The listing builds one solid part. Answer for the finished solid, in the listing's coordinates (mm). Give positions to 0.01 mm unless a question says otherwise; leave off trailing zeros. Write each loop counter-clockwise with the first axis right and the second up, starting at its lowest first coordinate (ties: lowest second). Pieces come first, ordered by that corner, then holes.
```python
from build123d import *

# Parameters (mm, degrees)
SKETCH1_W                        = 44.45
SKETCH1_H                        = 44.45
SKETCH1_W_2                      = 38.1
SKETCH1_H_2                      = 38.1
BOSS_EXTRUDE1_DEPTH              = 1936.75
F_17_64_0_26563_DIAMETER_HOLE1_D = 6.747002


with BuildPart() as part:
    # Sketch1 → Boss-Extrude1 (new body)
    with BuildSketch(Plane(origin=(0, 0, 0), x_dir=(0, 0, -1), z_dir=(1, 0, 0))):
        with Locations((22.225, 22.225)):
            Rectangle(SKETCH1_W, SKETCH1_H)
        with Locations((22.225, 22.225)):
            Rectangle(SKETCH1_W_2, SKETCH1_H_2, mode=Mode.SUBTRACT)
    extrude(amount=BOSS_EXTRUDE1_DEPTH)

    # 17/64 (0.26563) Diameter Hole1 (through all)
    with Locations(Plane.XY):
        with Locations((850.9, 22.225), (1085.85, 22.225)):
            Hole(F_17_64_0_26563_DIAMETER_HOLE1_D / 2)


solid = part.part
```
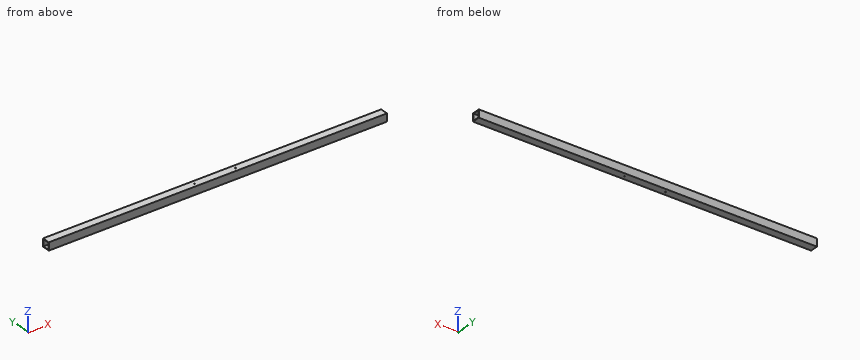
Item 1: Consider probe 1 along Y at (x, z) = (1546.5, -5.5) (3 decimals); probe 2 along Y at (x, z) = (1085.85, -1.6); probe 3 along Z at (x, y) = (226, 23) (3 decimals). Determine where each line is inside the solid, lowest interval first.
Conclusion:
probe 1: y = 0 to 3.175, 41.275 to 44.45
probe 2: y = 0 to 18.85, 25.6 to 44.45
probe 3: z = -44.45 to -41.275, -3.175 to 0
Item 2: A cutting plane is placed at C-C, the plane x = 1197.5. Give the vertices of the cut face in (y, z) (3 decimals), plus the area to 3 significant figures.
Conclusion:
outline: (0, -44.45) - (44.45, -44.45) - (44.45, 0) - (0, 0) - close; hole (3.175, -41.275) - (41.275, -41.275) - (41.275, -3.175) - (3.175, -3.175) - close
area: 524 mm2
Item 3: A cutting plane is placed at B-B, the plane y = 11. Give the vertices of the cut face in (x, z) (3 decimals).
Conclusion:
outline: (0, -44.45) - (1936.75, -44.45) - (1936.75, -41.275) - (0, -41.275) - close; (0, -3.175) - (1936.75, -3.175) - (1936.75, 0) - (0, 0) - close
Item 4: A cutting plane is placed at A-A, the plane z = -30. Give the vertices of the cut face in (x, y) (3 decimals).
Conclusion:
outline: (0, 0) - (1936.75, 0) - (1936.75, 3.175) - (0, 3.175) - close; (0, 41.275) - (1936.75, 41.275) - (1936.75, 44.45) - (0, 44.45) - close
